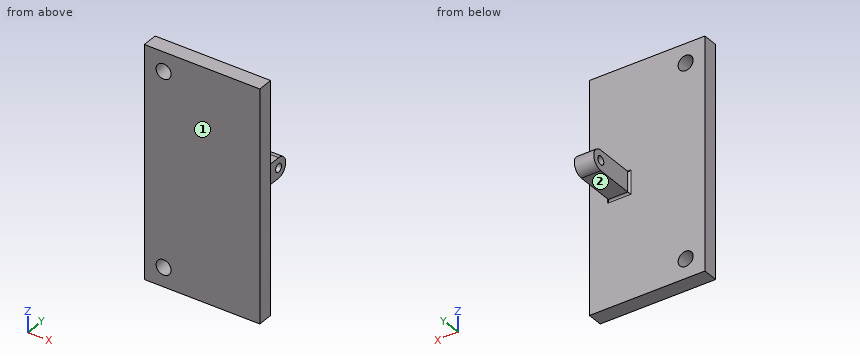
from build123d import *

# Parameters (mm, degrees)
BOSS_EXTRUDE1_DEPTH                    = 50.5
TAP_DRILL_FOR_M24X2_0_TAP1_D           = 22
TAP_DRILL_FOR_M24X2_0_TAP1_CSINK_D     = 22.05
TAP_DRILL_FOR_M24X2_0_TAP1_CSINK_ANGLE = 90
BOSS_EXTRUDE2_DEPTH                    = 40
FILLET1_R                              = 5
TAP_DRILL_FOR_M42X3_0_TAP1_D           = 39
TAP_DRILL_FOR_M42X3_0_TAP1_CSINK_D     = 39.05
TAP_DRILL_FOR_M42X3_0_TAP1_CSINK_ANGLE = 90


with BuildPart() as part:
    # Sketch1 → Boss-Extrude1 (new body)
    with BuildSketch(Plane(origin=(0, 0, 0), x_dir=(0, 0, -1), z_dir=(1, 0, 0))):
        with BuildLine():
            Line((-26.25, 0), (-26.25, -105))
            Line((-26.25, -105), (26.25, -105))
            Line((26.25, -105), (26.25, 0))
            ThreePointArc((26.25, 0), (0, 26.25), (-26.25, 0))
        make_face()
    extrude(amount=BOSS_EXTRUDE1_DEPTH)

    # Tap Drill for M24x2.0 Tap1 (through all)
    with Locations(Plane.ZY):
        with Locations((0, 0)):
            CounterSinkHole(TAP_DRILL_FOR_M24X2_0_TAP1_D / 2, TAP_DRILL_FOR_M24X2_0_TAP1_CSINK_D / 2, counter_sink_angle=TAP_DRILL_FOR_M24X2_0_TAP1_CSINK_ANGLE)

    # Sketch6 → Boss-Extrude2 (add)
    with BuildSketch(Plane.XZ.offset(105)):
        Polygon((103, 0), (103, 300), (-197, 300), (-197, -300), (103, -300), align=None)
    extrude(amount=BOSS_EXTRUDE2_DEPTH)

    # Fillet1
    fillet1_edges = [part.edges().sort_by_distance(p)[0] for p in [
        (50.5, -105, 0),
        (0, -105, 0),
        (25.25, -105, -26.25),
        (25.25, -105, 26.25),
    ]]
    fillet(fillet1_edges, radius=FILLET1_R)

    # Tap Drill for M42x3.0 Tap1 (through all)
    with Locations(Plane(origin=(0, -105, 0), x_dir=(1, 0, 0), z_dir=(0, 1, 0))):
        with Locations((-147, 250), (-147, -250)):
            CounterSinkHole(TAP_DRILL_FOR_M42X3_0_TAP1_D / 2, TAP_DRILL_FOR_M42X3_0_TAP1_CSINK_D / 2, counter_sink_angle=TAP_DRILL_FOR_M42X3_0_TAP1_CSINK_ANGLE)


solid = part.part
Work out the finished part from the listing and answer in its coordinate system (mm). Face numbers are marked on the shaded views. A direction names the side the tool comes from. Coordinates: 2 decimals unless noted, no trailing zeros. Write each loop counter-clockwise with the first axis right and the second up, starting at its lowest first coordinate (ties: lowest second). Pieces come first, ordered by that corner, then holes. Notation, with made-up numbers: M 85.25,37.5 L 132.25,37.5 A19 ccw 132.25,57.5 Z; hole C 74.5,40.25 d7. An arc over 180 degrees is marked long. Use one line per item in the form item = value. Start each with the question number.
1. Straight lines are drawn through the part: probe 1 along Z at (x, y) = (-147, -116); probe 2 along X at (y, z) = (-125, -250); probe 3 along Y at (x, z) = (39, 0). For each, find the intervals that lie inside material, in ascending order. Write a range as from..to.
2. The part is cut by section C-C (z = 143). Give the vertices of the cut face in (x, y).
3. A tool of negligible diameter and unlimited length cuts with its end or side. For the marked faces 1 and 2, from which of +Z, -Z, +X, -X, +Y, -Y can it reach the whole face along a straight path? Write none if from no direction.
4. The part is cut by section B-B (z = 0). Give the vertices of the cut face in (x, y) (3 decimals), plus the area to 3 significant figures.
5. The part is cut by section A-A (z = 250). Give the vertices of the cut face in (x, y) (3 decimals).
6. The part is cut by section D-D (y = -80.5). Give the vertices of the cut face in (x, z).
7. Each of these flat-tipped pins is pushed along its axis until it touches: P1, Ø12, axis at x = 36.5, y = -101, coming from the -Z side; P2, Ø4, axis at x = -144.5, z = -66, coming from the +Y side; P3, Ø13, axis at y = 0, z = 0, coming from the +X side. Where does it stop, or does it pass through?
Evaluation:
q1.probe_1 = -300..-269.5, -230.5..230.5, 269.5..300
q1.probe_2 = -197..-166.5, -127.5..103
q1.probe_3 = -145..-11, 11..26.25
q2.outline = M -197,-145 L 103,-145 L 103,-105 L -197,-105 Z
q3.face_1 = +Z, -Z, +X, -X, -Y
q3.face_2 = -Z, +X, -X, +Y
q4.outline = M -197,-145 L 103,-145 L 103,-105 L 55.5,-105 A5 cw 50.5,-100 L 50.5,-11 L 0.025,-11 L 0,-11.025 L 0,-100 A5 cw -5,-105 L -197,-105 Z; M 0,11.025 L 0.025,11 L 50.5,11 L 50.5,26.25 L 0,26.25 Z
q4.area = 17,500 mm^2
q5.outline = M -197,-145 L -166.5,-145 L -166.5,-105.025 L -166.525,-105 L -197,-105 Z; M -127.5,-145 L 103,-145 L 103,-105 L -127.475,-105 L -127.5,-105.025 Z
q6.outline = M 0,-26.25 L 50.5,-26.25 L 50.5,26.25 L 0,26.25 Z
q7.P1 = -300
q7.P2 = -105
q7.P3 = through
